Source: three-view drawing plus pictorial views. Frame: mm from the lowest corner of the part. Give positions to 0.01 mm unless a question says otherwise; leave off trailing zeros. Loops run counter-clockwise (first coordinate to the right, second up) from the corner with the lowest first, then second, coordinate; pieces in that order, holes last. Notation, with made-up numbers: M 15.25,72 L 28.25,72 A23 cw 28.25,104 Z; hole C -15,56 d9. An arc over 180 degrees is marked long. Answer as a JSON object with one key per item and string values. Group by question number.
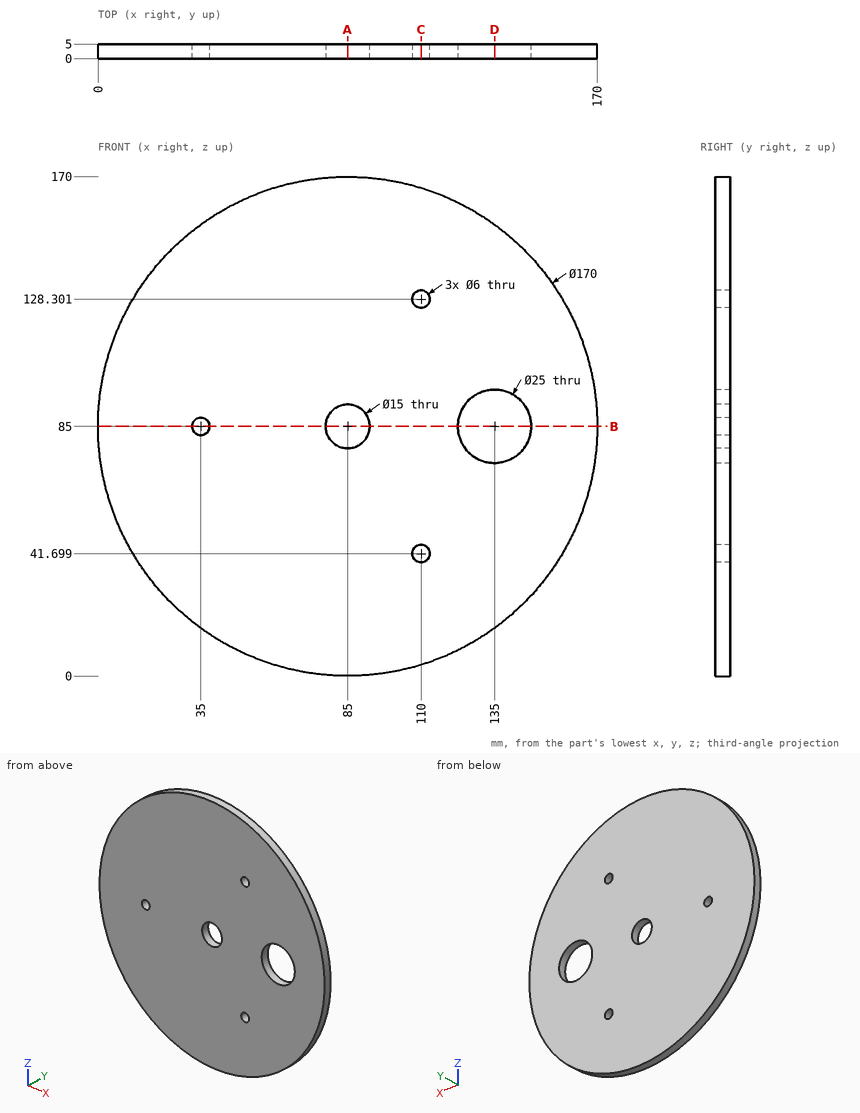
1. Material intervals for L1, parallel to X at y = 1.55, z = 83 (1 decimal); L2, parallel to Z at x = 110, y = 1.1; L3, parallel to Z at x = 85, y = 1.65, sorted ascending.
2. First-contact query: P1, Ø1.5, axis at x = 82, y = 2.5, coming from the +Z side; P2, Ø3, axis at x = 119, y = 0.5, coming from the +Z side. Flat tips, straight axial feed; report the tip coordinate or a pass-through.
3. Section A-A (x = 85). Output: boundary loops of the cut face in (y, z).
4. Section D-D (x = 135). Output: boundary loops of the cut face in (y, z).
5. Section B-B (z = 85). Output: boundary loops of the cut face in (x, y), then the cut area to 3 significant figures.
6. Section C-C (x = 110). Output: boundary loops of the cut face in (y, z).
Geometry results:
{
 "1": {"L1": "0 to 32.8, 37.2 to 77.8, 92.2 to 122.7, 147.3 to 170", "L2": "3.76 to 38.7, 44.7 to 125.3, 131.3 to 166.24", "L3": "0 to 77.5, 92.5 to 170"},
 "2": {"P1": "z = 169.97", "P2": "z = 163.54"},
 "3": {"outline": "M 0,0 L 5,0 L 5,77.5 L 0,77.5 Z; M 0,92.5 L 5,92.5 L 5,170 L 0,170 Z"},
 "4": {"outline": "M 0,16.26 L 5,16.26 L 5,72.5 L 0,72.5 Z; M 0,97.5 L 5,97.5 L 5,153.74 L 0,153.74 Z"},
 "5": {"outline": "M 0,0 L 32,0 L 32,5 L 0,5 Z; M 38,0 L 77.5,0 L 77.5,5 L 38,5 Z; M 92.5,0 L 122.5,0 L 122.5,5 L 92.5,5 Z; M 147.5,0 L 170,0 L 170,5 L 147.5,5 Z", "area": "620 mm2"},
 "6": {"outline": "M 0,3.76 L 5,3.76 L 5,38.7 L 0,38.7 Z; M 0,44.7 L 5,44.7 L 5,125.3 L 0,125.3 Z; M 0,131.3 L 5,131.3 L 5,166.24 L 0,166.24 Z"}
}
